The listing builds one solid part. Answer for the finished solid, in the listing's coordinates (mm). A direction names the side the tool comes from. Give positions to 0.01 mm unless a question says otherwise; leave off trailing zeros. Order: outer loops, then holes, each group sorted by start corner. A loop starts at its lowest first (then second) coordinate and runs counter-clockwise, first axis right, second up. Notation, with made-up numbers: (37, 64.5) - (68, 64.5) arc R33 ccw to (68, 100.5) - close; hole circle Ø11 at (53, 11). An arc over 180 degrees is marked (long way). Answer as CSV lines item,"result". Start each with the question number.
1. Section D-D on y = -7 is taken. Give the vertices of the cut face in (x, z), and give its area (3 significant figures).
2. Section A-A on x = -80 is taken. Give the vertices of the cut face in (y, z).
3. Section C-C on x = -13 is taken. Give the vertices of the cut face in (y, z).
4. Which of the six approach directions +Z, -Z, +X, -X, +Y, -Y give full straight-line access (tool end or side, diameter ignored) to faces 4 (the flat face through (38, -13, -5)), 5 (the cylindrical face through (0.488, -2.535, -77.804))?
5. Determine the mould class of faces 1 (the conical face through (22.476, -14.514, -1.644)), 2 (the cylindrical face through (-82.08, -2.53, 0.86)), 3 (the flat face through (1, 0, -1)) for opening direction Z: +Z half, -Z half, draft (parallel to the pull), parting line (faces both ways), or undercut.
6. Consider line 1 along X through (y, z) = (-4.75, 58); line 2 along Y through (x, z) = (-71.5, -9); line 3 along Z through (x, y) = (35, -14.45) (3 decimals). Determine where each line is inside the solid, lowest interval first. Write a range as [from, to].
7. Flat-ended cylindrical pins translate along their axes: pin 1 (4 mm diameter, centred on x = -16.5, y = -3.5, fed in from -Z); pin 2 (4 mm diameter, centred on x = 53.5, y = -5.5, fed in from -Z); pin 3 (3 mm diameter, centred on x = 37.5, z = 1.5, fed in from +Y); pin 4 (7 mm diameter, centred on x = -56.57, z = -56.57, fed in from +Y). Find the tip coordinate at first contact, or state that the pin passes through.
8. Section B-B on z = -80 is taken. Give the vertices of the cut face in (x, y), and give its area (3 significant figures).
from build123d import *

# Parameters (mm, degrees)
EXTRUDE_START      = -5
SKETCH_6_R         = 85
SKETCH_6_R_2       = 25
EXTRUDE_1041_DEPTH = 5
HOLE_WIZARD_M4_8_D = 4.5


with BuildPart() as part:
    # 草图2 → Revolve 925 (revolve)
    with BuildSketch(Plane.XY, mode=Mode.PRIVATE) as revolve_925_sk:
        Polygon((32, -15), (32, -14), (29.75, -14), (29.75, -13), (22.75, -13), (10, 0), (10, -5), (23, -15), align=None)
    revolve(revolve_925_sk.sketch.rotate(Axis((35, 1.713666668, 0), (0, -1, 0)), 270), axis=Axis((35, 1.713666668, 0), (0, -1, 0)))

    # 草图6 → Extrude 1041 (add)
    with BuildSketch(Plane(origin=(0, 0, 0), x_dir=(1, 0, 0), z_dir=(0, 1, 0)).offset(EXTRUDE_START)):
        with Locations(Location((0, 0, 0), (0, 0, 270))):
            Circle(SKETCH_6_R)
        with Locations((35, 0)):
            Circle(SKETCH_6_R_2, mode=Mode.SUBTRACT)
    extrude(amount=EXTRUDE_1041_DEPTH)

    # M4*8 固定孔 (through all)
    with Locations(Plane(origin=(0, 0, 0), x_dir=(1, 0, 0), z_dir=(0, 1, 0))):
        with Locations((80, 0), (-80, 0), (-56.568542495, 56.568542495), (0, 80), (56.568542495, -56.568542495), (0, -80), (-56.568542495, -56.568542495), (56.568542495, 56.568542495)):
            Hole(HOLE_WIZARD_M4_8_D / 2)


solid = part.part
Checks:
1,outline,"circle Ø44.8 at (35, 0); hole circle Ø36.27 at (35, 0)"
1,area,"543 mm²"
2,outline,"(-5, -28.72) - (0, -28.72) - (0, -2.25) - (-5, -2.25) - close; (-5, 2.25) - (0, 2.25) - (0, 28.72) - (-5, 28.72) - close"
3,outline,"(-5, -84) - (0, -84) - (0, 84) - (-5, 84) - close"
4,face 4,"+Y"
4,face 5,"+Y, -Y"
5,face 1,"parting line"
5,face 2,"undercut"
5,face 3,"draft"
6,line 1,"x = [-62.14, -58.3], [-54.83, 54.83], [58.3, 62.14]"
6,line 2,"y = [-5, 0]"
6,line 3,"z = [-12.715, -3], [3, 12.715]"
7,pin 1,"stops at z = -83.75"
7,pin 2,"stops at z = -67.57"
7,pin 3,"stops at y = -14"
7,pin 4,"stops at y = 0"
8,outline,"(-28.72, -5) - (-2.25, -5) - (-2.25, 0) - (-28.72, 0) - close; (2.25, -5) - (28.72, -5) - (28.72, 0) - (2.25, 0) - close"
8,area,"265 mm²"
